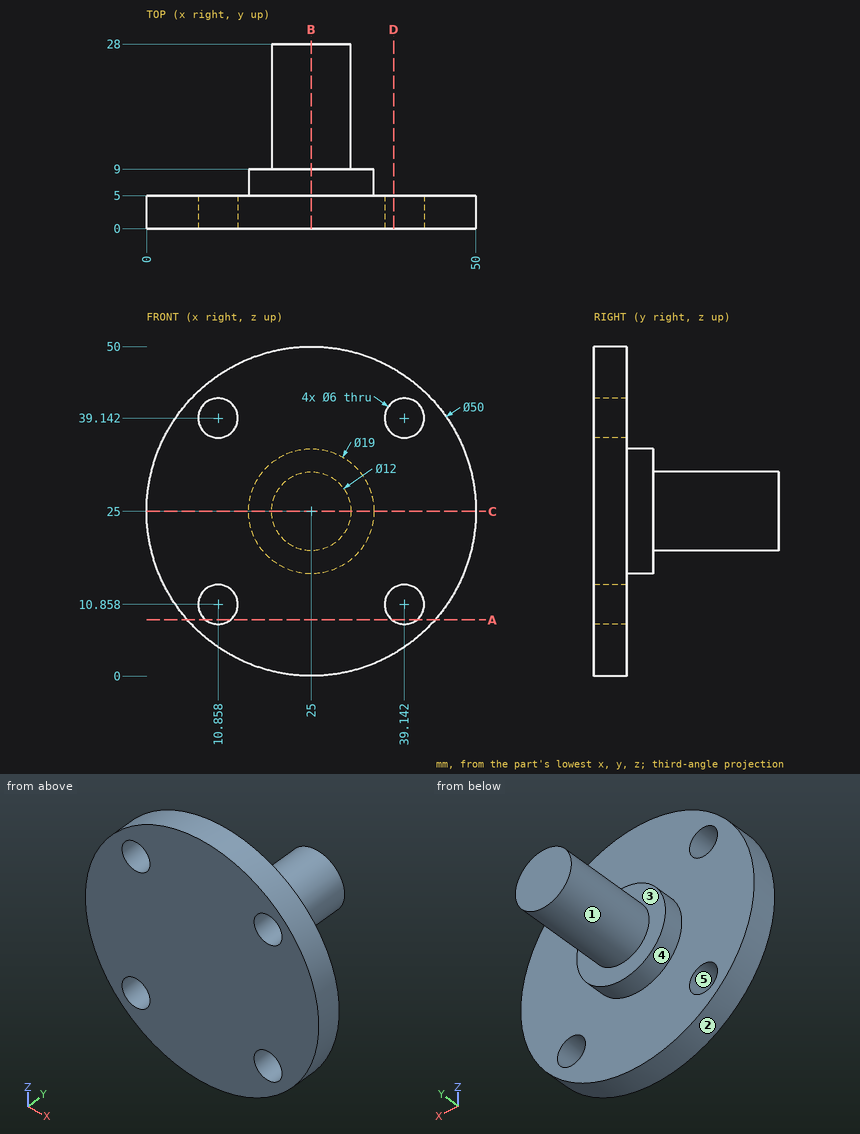
Part print with two shaded views. Sizes in mm from the minimum x, y, z corner. A direction names the side the tool comes from. Coordinates: 2 decimals unless noted, no trailing zeros. Order: outer loops, then holes, each group sorted by start corner. A loop starts at its lowest first (then second) coordinate and runs counter-clockwise, first axis right, second up. Notation, with made-up numbers: (48.25, 76) - (104.25, 76) arc R14 ccw to (104.25, 92) - close; hole circle Ø4 at (84.25, 59). An arc over 180 degrees is marked (long way). Answer in a Markdown table with one row per item.
1. Slice it at A-A, the plane z = 8.5. List the corners of the cut face in (x, y).
Answer:
| item | result |
|---|---|
| outline | (6.22, 0) - (9, 0) - (9, 5) - (6.22, 5) - close; (12.71, 0) - (37.29, 0) - (37.29, 5) - (12.71, 5) - close; (41, 0) - (43.78, 0) - (43.78, 5) - (41, 5) - close |
2. Drill centre lines: L1, parallel to Y at x = 16.5, z = 15; L2, parallel to X at y = 24.75, z = 25; L3, parallel to Z at x = 32, y = 1.5. Where is each one in solid material? Low to high. Write a range as from..to.
Answer:
| item | result |
|---|---|
| L1 | 0..5 |
| L2 | 19..31 |
| L3 | 1..49 |
3. Slice it at B-B, the plane x = 25. List the corners of the cut face in (y, z).
Answer:
| item | result |
|---|---|
| outline | (0, 0) - (5, 0) - (5, 15.5) - (9, 15.5) - (9, 19) - (28, 19) - (28, 31) - (9, 31) - (9, 34.5) - (5, 34.5) - (5, 50) - (0, 50) - close |
4. 3-axis set-ups, long thin cutter, end or side, ignore diameter. For the marked faces 1 and 2: which of +Z, -Z, +X, -X, +Y, -Y reach the whole face in a straight line?
Answer:
| item | result |
|---|---|
| face 1 | +Y |
| face 2 | +Y, -Y |
5. Slice it at D-D, the plane x = 37.5. List the corners of the cut face in (y, z), then the cut area to 3 significant figures.
Answer:
| item | result |
|---|---|
| outline | (0, 3.35) - (5, 3.35) - (5, 8.35) - (0, 8.35) - close; (0, 13.37) - (5, 13.37) - (5, 36.63) - (0, 36.63) - close; (0, 41.65) - (5, 41.65) - (5, 46.65) - (0, 46.65) - close |
| area | 166 mm² |
6. Flat gauge pins, fed straight in: P1, Ø8, axis at x = 39.14, z = 10.86, coming from the +Y side; P2, Ø4, axis at x = 23, z = 34.5, coming from the +Y side; P3, Ø5, axis at x = 30, y = 5.5, coming from the +Z side. Where does each tip first touch, or does it go through?
Answer:
| item | result |
|---|---|
| P1 | y = 5 |
| P2 | y = 9 |
| P3 | z = 49.87 |
7. Pull direction Z, two halves, no side cores. Call the marked faces 3, 4 and 5: +Z half, -Z half, draft (parallel to the pull), parting line (faces both ways), or undercut.
Answer:
| item | result |
|---|---|
| face 3 | draft |
| face 4 | parting line |
| face 5 | undercut |
8. Slice it at C-C, the plane z = 25. List the corners of the cut face in (x, y).
Answer:
| item | result |
|---|---|
| outline | (0, 0) - (50, 0) - (50, 5) - (34.5, 5) - (34.5, 9) - (31, 9) - (31, 28) - (19, 28) - (19, 9) - (15.5, 9) - (15.5, 5) - (0, 5) - close |
